Study the drawing (mm; zero at the part's minimum x, y, z) and answer. Give positions to 0.01 mm unless a question says otherwise; leave off trailing zeros. Loops run counter-clockwise (first coordinate to the right, second up) from the corner with the lowest first, then second, coordinate; pieces in that order, holes last. Notation, with made-up numbers: M -23,-35 L -1,-35 A10 cw -1,-16 Z; hole C 43.25,-36.75 d7. An arc over 180 degrees is marked long. Return JSON: item names as keys, results as strings.
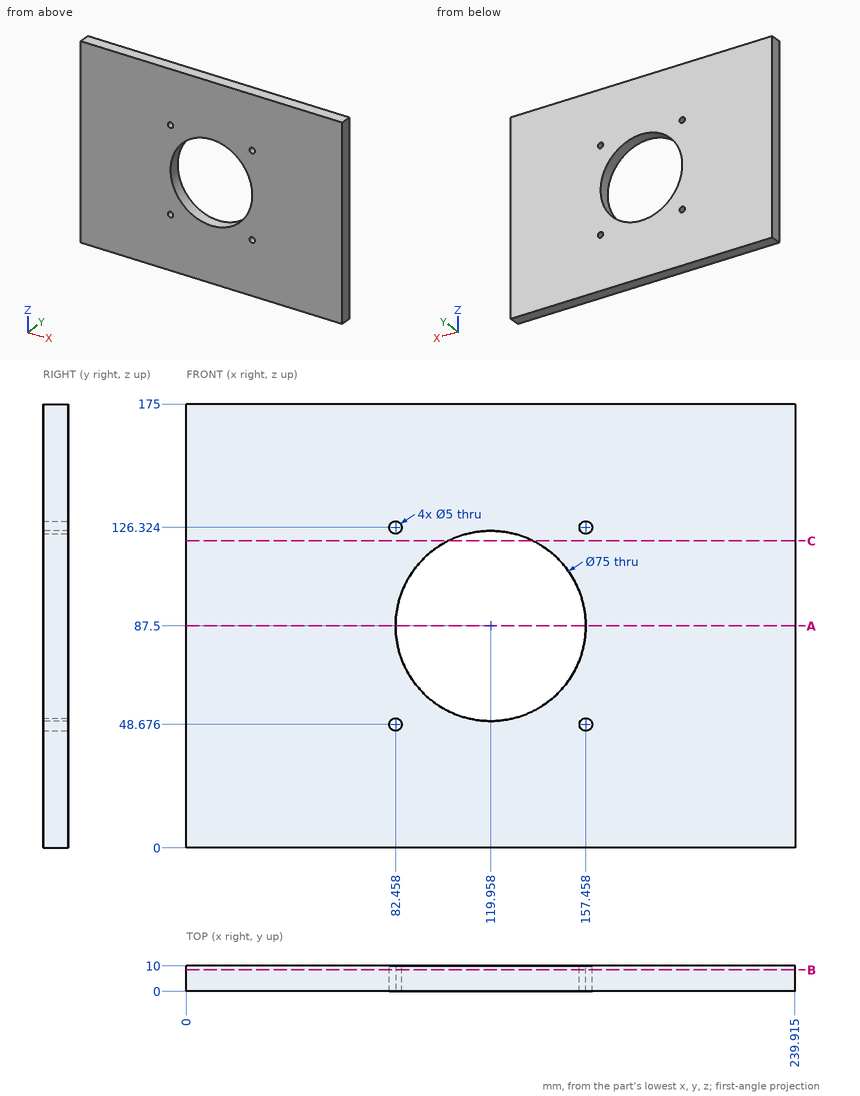
(1) The part is cut by section B-B (y = 8.5). Determine the outline of the cut face in (x, z) (1 decimal), and give its area (3 significant figures).
Values follow:
{"outline": "M 0,0 L 239.9,0 L 239.9,175 L 0,175 Z; hole C 82.5,48.7 d5; hole C 82.5,126.3 d5; hole C 120,87.5 d75; hole C 157.5,48.7 d5; hole C 157.5,126.3 d5", "area": "37,500 mm²"}
(2) The part is cut by section C-C (z = 121). Determine the outline of the cut face in (x, y) (1 decimal), and give its area (3 significant figures).
Values follow:
{"outline": "M 0,0 L 103.1,0 L 103.1,10 L 0,10 Z; M 136.8,0 L 239.9,0 L 239.9,10 L 136.8,10 Z", "area": "2,060 mm²"}
(3) The part is cut by section A-A (z = 87.5). Determine the outline of the cut face in (x, y) (1 decimal).
Values follow:
{"outline": "M 0,0 L 82.5,0 L 82.5,10 L 0,10 Z; M 157.5,0 L 239.9,0 L 239.9,10 L 157.5,10 Z"}
(4) Straight lines are drawn through the part: line 1 along X through (y, z) = (8, 49) (1 decimal); line 2 along X through (y, z) = (1, 46.5) (1 decimal); line 3 along X through (y, z) = (7, 87.5) (1 decimal). For each, find the intervals that lie inside material, in ascending order.
Values follow:
{"line 1": "0 to 80, 84.9 to 155, 159.9 to 239.9", "line 2": "0 to 81.2, 83.7 to 156.2, 158.7 to 239.9", "line 3": "0 to 82.5, 157.5 to 239.9"}
